from build123d import *

# Parameters (mm, degrees)
SKETCH_1_R          = 5
EXTRUDE_1_DEPTH     = 4
SKETCH_2_R          = 5
EXTRUDE_2_DEPTH     = 10
CUT_EXTRUDE_2_DEPTH = 170.257200733
CHAMFER_1_SIZE      = 37.320508076
CHAMFER_1_SIZE_2    = 10
EXTRUDE_3_DEPTH     = 2
SKETCH_6_W          = 2
SKETCH_6_H          = 48
CUT_EXTRUDE_4_DEPTH = 170.54055562
SKETCH_7_R          = 1.45
CUT_EXTRUDE_5_DEPTH = 170.857764694


with BuildPart() as part:
    # 스케치1 → 보스-돌출1 (new body)
    with BuildSketch(Plane(origin=(0, 0, 0), x_dir=(1, 0, 0), z_dir=(0, 1, 0))):
        with BuildLine():
            ThreePointArc((18, 150), (0, 168), (-18, 150))
            Line((-18, 150), (-18, 0))
            ThreePointArc((-18, 0), (0, -18), (18, 0))
            Line((18, 0), (18, 150))
        make_face()
        with BuildLine():
            ThreePointArc((-15, -1.2), (-16.2, 0), (-15, 1.2))
            Line((-15, 1.2), (-4.85386444, 1.2))
            ThreePointArc((-4.85386444, 1.2), (-3.535533906, 3.535533906), (-1.2, 4.85386444))
            Line((-1.2, 4.85386444), (-1.2, 15))
            ThreePointArc((-1.2, 15), (0, 16.2), (1.2, 15))
            Line((1.2, 15), (1.2, 4.85386444))
            ThreePointArc((1.2, 4.85386444), (3.535533906, 3.535533906), (4.85386444, 1.2))
            Line((4.85386444, 1.2), (15, 1.2))
            ThreePointArc((15, 1.2), (16.2, 0), (15, -1.2))
            Line((15, -1.2), (4.85386444, -1.2))
            ThreePointArc((4.85386444, -1.2), (3.535533906, -3.535533906), (1.2, -4.85386444))
            Line((1.2, -4.85386444), (1.2, -15))
            ThreePointArc((1.2, -15), (0, -16.2), (-1.2, -15))
            Line((-1.2, -15), (-1.2, -4.85386444))
            ThreePointArc((-1.2, -4.85386444), (-3.535533906, -3.535533906), (-4.85386444, -1.2))
            Line((-4.85386444, -1.2), (-15, -1.2))
        make_face(mode=Mode.SUBTRACT)
        with Locations(Location((0, 150, 0), (0, 0, 270))):
            Circle(SKETCH_1_R, mode=Mode.SUBTRACT)
    extrude(amount=EXTRUDE_1_DEPTH)

    # 스케치2 → 보스-돌출2 (add)
    with BuildSketch(Plane(origin=(0, 4, 0), x_dir=(1, 0, 0), z_dir=(0, 1, 0))):
        with BuildLine():
            Line((-18, 100), (18, 100))
            Line((18, 100), (18, 150))
            ThreePointArc((18, 150), (0, 168), (-18, 150))
            Line((-18, 150), (-18, 100))
        make_face()
        with Locations(Location((0, 150, 0), (0, 0, 270))):
            Circle(SKETCH_2_R, mode=Mode.SUBTRACT)
    extrude(amount=EXTRUDE_2_DEPTH)

    # 스케치4 → 컷-돌출2 (cut, symmetric)
    with BuildSketch(Plane(origin=(0, 4, 0), x_dir=(1, 0, 0), z_dir=(0, 1, 0))):
        with BuildLine():
            Line((-10.5, 29.047375097), (-10.5, 112.009618943))
            Line((-10.5, 112.009618943), (-18, 125))
            Line((-18, 125), (-18, 0))
            ThreePointArc((-18, 0), (-16.094750193, 15), (-10.5, 29.047375097))
        make_face()
    cut_extrude_2 = extrude(amount=CUT_EXTRUDE_2_DEPTH, both=True, mode=Mode.SUBTRACT)

    # 대칭 복사1: 컷-돌출2 across plane
    add(cut_extrude_2.mirror(Plane(origin=(0, 0, 0), x_dir=(0, 0, 1), z_dir=(1, 0, 0))), mode=Mode.SUBTRACT)

    # 모따기1
    # the kernel refuses this chamfer: 37.320508076, 10 mm, written as the material it takes off along each edge
    with BuildSketch(Plane(origin=(-107.410968331, 14, -100), x_dir=(0, 0.009967146577156314, -0.9999503267608394), z_dir=(1, 0, 0))) as chamfer_1_piece_1_section:
        Polygon((CHAMFER_1_SIZE * 0.999950326753, -CHAMFER_1_SIZE * 0.00996714657707), (-CHAMFER_1_SIZE_2 * 0.00996714657716, -CHAMFER_1_SIZE_2 * 0.999950326761), (0, 0), align=None)
    chamfer_1_piece_1 = extrude(amount=214.821936662, mode=Mode.PRIVATE)
    chamfer_1_piece_1 = split(chamfer_1_piece_1, bisect_by=Plane(origin=(0, 4, -113.026597383), z_dir=(0, 1, 0)), keep=Keep.TOP, mode=Mode.PRIVATE)
    add(chamfer_1_piece_1, mode=Mode.SUBTRACT)

    # 스케치5 → 보스-돌출3 (add, symmetric)
    with BuildSketch(Plane(origin=(0, 0, 0), x_dir=(0, 0, -1), z_dir=(1, 0, 0))):
        with BuildLine():
            Line((25, 4), (125, 4))
            ThreePointArc((125, 4), (75, 9.051025722), (25, 4))
        make_face()
    extrude(amount=EXTRUDE_3_DEPTH, both=True)

    # 스케치6 → 컷-돌출4 (cut, through all)
    with BuildSketch(Plane(origin=(0, 14, 0), x_dir=(1, 0, 0), z_dir=(0, 1, 0))):
        with BuildLine():
            Line((-3, 167.748239349), (-3, 160.748239349))
            ThreePointArc((-3, 160.748239349), (-8.888245975, 156.74712773), (-11.159061301, 150))
            Line((-11.159061301, 150), (-11.159061301, 113.151146601))
            Line((-11.159061301, 113.151146601), (-22.159061301, 113.151146601))
            Line((-22.159061301, 113.151146601), (-22.159061301, 167.748239349))
            Line((-22.159061301, 167.748239349), (-3, 167.748239349))
        make_face()
        with BuildLine():
            Line((22.159061301, 167.748239349), (3, 167.748239349))
            Line((3, 167.748239349), (3, 160.748239349))
            ThreePointArc((3, 160.748239349), (8.888245975, 156.74712773), (11.159061301, 150))
            Line((11.159061301, 150), (11.159061301, 113.151146601))
            Line((11.159061301, 113.151146601), (22.159061301, 113.151146601))
            Line((22.159061301, 113.151146601), (22.159061301, 167.748239349))
        make_face()
        with Locations((0, 168)):
            Rectangle(SKETCH_6_W, SKETCH_6_H)
    extrude(amount=-CUT_EXTRUDE_4_DEPTH, mode=Mode.SUBTRACT)

    # 스케치7 → 컷-돌출5 (cut, through all)
    with BuildSketch(Plane(origin=(3, 0, 0), x_dir=(0, 0, -1), z_dir=(1, 0, 0))):
        with Locations((164.248239349, 11)):
            Circle(SKETCH_7_R)
        with Locations((164.248239349, 3)):
            Circle(SKETCH_7_R)
    extrude(amount=-CUT_EXTRUDE_5_DEPTH, mode=Mode.SUBTRACT)


solid = part.part
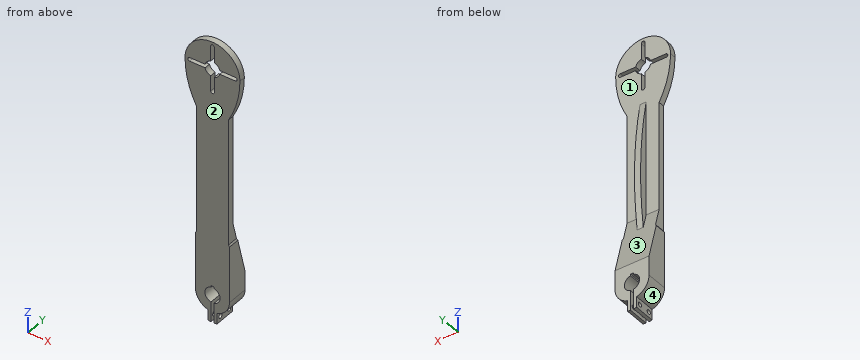
Design review of the part built by this model. Coordinates are the model's own, in mm. Face numbers are marked on the shaded views. A direction names the side the tool comes from. Coordinates: 2 decimals unless noted, no trailing zeros. Write each loop counter-clockwise with the first axis right and the second up, starting at its lowest first coordinate (ties: lowest second). Pieces come first, ordered by that corner, then holes. Notation, with made-up numbers: (32.5, -15) -> (67.5, -15) arc R11 cw to (67.5, 1) -> close; hole circle Ø9 at (-28, -32). An arc over 180 degrees is marked (long way). Write each question's results on one line, items separated by ' | '. Start each with the question number.
(1) Take a section at A-A on x = 8.5. Write out the cut boundary in (y, z).
(2) For line 1 along X through (y, z) = (4.5, -28.5); line 2 along X through (y, z) = (1.5, -142.5); line 3 along Y through (x, z) = (-10, 8), list the stretches that pass through material, from the lowest coordinate up. Write a range as from..to.
(3) Clearance check with flat-ended pins moving along their axes: P1, Ø4.5, axis at x = 9.5, y = 2, coming from the +Z side; P2, Ø2, axis at y = 1, z = 11, coming from the -X side; P3, Ø5, axis at x = 5, y = 6, coming from the +Z side; P4, Ø2, axis at x = -13, z = -117.5, coming from the -Y side. State where each tip first meets the part, or that it passes through.
(4) The part is to be moulded in two halves that separate along X. For the marked faces 3 and 4, say which applies: pulls with the +X half, pulls with the -X half, needs draft (parallel to the pull), parting line crosses it, or undercut.
(5) Take a section at B-B on z = -37.5. Write out the cut boundary in (x, y), and give its area (3 significant figures).
(6) Tool access review of the marked faces 1 and 2: name each direction out of +Z, -Z, +X, -X, +Y, -Y from which nothing blocks a thin tool from reaching the whole face with its end or side.
Results found:
1) outline: (0, -157.23) -> (14, -157.23) -> (14, -137.32) -> (4, -100) -> (4, -1.2) -> (0, -1.2) -> close; (0, 1.2) -> (4, 1.2) -> (4, 15.87) -> (0, 15.87) -> close
2) line 1: x = -2..2 | line 2: x = -11.16..11.16 | line 3: y = 0..4
3) P1: stops at z = 16.48 | P2: stops at x = -14.97 | P3: stops at z = 17.66 | P4: passes through
4) face 3: needs draft | face 4: pulls with the -X half
5) outline: (-10.5, 0) -> (10.5, 0) -> (10.5, 4) -> (2, 4) -> (2, 6.22) -> (-2, 6.22) -> (-2, 4) -> (-10.5, 4) -> close | area: 92.9 mm2
6) face 1: +Z, +Y | face 2: +Z, -Z, +X, -X, -Y
